The model under review builds one solid part; all positions refer to its coordinate system, in mm. Face numbers are marked on the shaded views. Round coordinates to 2 decimals unless told otherwise and drop trailing zeros. Order: outer loops, then holes, each group sorted by start corner. A loop starts at its lowest first (then second) coordinate and runs counter-clockwise, first axis right, second up. Notation, with made-up numbers: M 45,13.5 L 71,13.5 A16 cw 71,29.5 Z; hole C -6,48.5 d8. An arc over 180 degrees is marked long. Use a Markdown table: item, result. Add a question column.
1. Insertion check: P1, Ø1.5, axis at x = 83, y = 10, coming from the +Z side; P2, Ø3, axis at x = 2, z = 5, coming from the +Y side; P3, Ø3, axis at y = 27.5, z = 6, coming from the -X side; P4, Ø1, axis at x = 97.5, y = 11.5, coming from the -Z side. Each pin has a flat end and moves straight along its axis. Give the tip position at first contact, or say it passes through.
2. Consider section A-A on z = 2.75. State the section outline as (x, y) points, then the cut area to 3 significant figures.
3. To check wall thickness, follow probe 1 along Y at (x, z) = (-2.9, 0.55) (3 decimals); probe 2 along Y at (x, z) = (137.1, 0.75); probe 3 along Y at (x, z) = (67, 3.5). State the ranges of each line that lie inside material, in increasing order.
4. The part is to be moulded in two halves that separate along X. For the marked faces 1 and 2, say which applies: +X half, -X half, draft (parallel to the pull), parting line (faces both ways), or undercut.
5. Consider section C-C on x = 104.5. State the section outline as (y, z) points.
6. Consider section D-D on y = 20. State the section outline as (x, z) points, then the cut area to 3 significant figures.
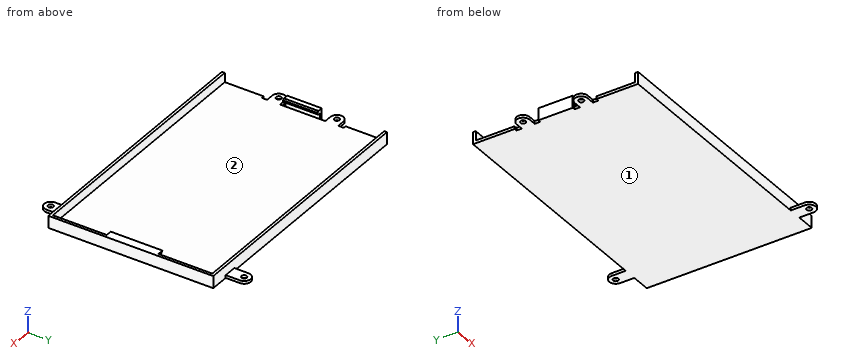
Autodesk Inventor part; units mm, degrees
ref_plane "YZ Plane" through (0, 0, 0) normal (1, 0, 0) x (0, 1, 0)
ref_plane "XZ Plane" through (0, 0, 0) normal (0, 1, 0) x (-1, 0, 0)
ref_plane "XY Plane" through (0, 0, 0) normal (0, 0, 1) x (1, 0, 0)
sketch "Sketch1" plane through (0, 0, 0) normal (0, 0, 1) x (1, 0, 0)
  line L0 (150.1, 1.6) -> (0, 1.6)
  line L1 (1.6, 24.1) -> (1.6, 71.6)
  line L2 (1.6, 24.1) -> (0, 24.1)
  line L3 (1.6, 47.85) -> (150.1, 47.85) construction
  line L4 (1.6, 71.6) -> (0, 71.6)
  line L5 (0, 71.6) -> (0, 94.1)
  line L6 (1.6, 30.975) -> (-2.9, 30.975) construction
  circle A0 centre (-2.9, 30.975) radius 1.5
  line L7 (-2.9, 27.225) -> (-2.9, 34.725) construction
  line L8 (-2.9, 27.225) -> (1.6, 27.225)
  line L9 (-2.9, 34.725) -> (1.6, 34.725)
  line L10 (1.6, 57.85) -> (0, 57.85)
  line L11 (0, 57.85) -> (0, 37.85)
  line L12 (0, 37.85) -> (1.6, 37.85)
  line L13 (0, 57.85) -> (0, 68.475) construction
  line L14 (0, 37.85) -> (0, 27.225) construction
  line L15 (0, 24.1) -> (0, 34.725) construction
  line L16 (151.7, 0) -> (0, 0)
  line L17 (151.7, 95.7) -> (0, 95.7)
  line L18 (0, 95.7) -> (0, 94.1)
  line L19 (0, 94.1) -> (150.1, 94.1)
  line L20 (137.1, 94.1) -> (137.1, 103.95) construction
  circle A1 centre (137.1, 103.95) radius 1.5
  arc A2 (140.85, 103.95) -> (133.35, 103.95) centre (137.1, 103.95) ccw
  line L21 (133.35, 103.95) -> (140.85, 103.95) construction
  line L22 (140.85, 103.95) -> (140.85, 95.7)
  line L23 (133.35, 103.95) -> (133.35, 95.7)
  line L24 (137.1, 1.6) -> (137.1, -8.25) construction
  circle A3 centre (137.1, -8.25) radius 1.5
  arc A4 (133.35, -8.25) -> (140.85, -8.25) centre (137.1, -8.25) ccw
  line L25 (133.35, -8.25) -> (140.85, -8.25) construction
  line L26 (140.85, -8.25) -> (140.85, 0)
  line L27 (133.35, -8.25) -> (133.35, 0)
  arc A5 (-2.9, 34.725) -> (-2.9, 27.225) centre (-2.9, 30.975) ccw
  line L28 (150.1, 94.1) -> (150.1, 1.6)
  line L29 (151.7, 0) -> (151.7, 95.7)
  line L30 (0, 24.1) -> (0, 0)
  line L31 (1.6, 64.725) -> (-2.9, 64.725) construction
  circle A6 centre (-2.9, 64.725) radius 1.5
  line L32 (-2.9, 68.475) -> (-2.9, 60.975) construction
  line L33 (1.6, 68.475) -> (-2.9, 68.475)
  line L34 (1.6, 60.975) -> (-2.9, 60.975)
  arc A7 (-2.9, 68.475) -> (-2.9, 60.975) centre (-2.9, 64.725) ccw
  point P0 (0, 0)
  dimension "d8" = 3
  dimension "d9" = 4.5
  dimension "d11" = 1.6
  dimension "d14" = 3
  dimension "d15" = 7.5
  dimension "d17" = 7.5
  dimension "d19" = 112.2
  dimension "d23" = 1.6
  dimension "d27" = 22.5
  dimension "d28" = 1.6
  dimension "d29" = 1.6
  dimension "d30" = 148.5
  dimension "d31" = 92.5
  dimension "d32" = 1.6
  dimension "d34" = 140
  dimension "d36" = 33.75
  dimension "d37" = 7.5
extrude "Extrusion1" add sketch "Sketch1" along normal blind 1.6
extrude "Extrusion2" add sketch "Sketch1" along normal blind 7 contours L28 L19 L18 L17 L29 L16 L30 L0 | L12 L11 L10 L1
sketch "Sketch2" plane through (150.1, 1.6, 1.6) normal (-1, 0, 0) x (0, 0, 1)
  line L0 (-1.6, -1.6) -> (-1.6, 94.1)
  line L1 (-1.6, 94.1) -> (5.4, 94.1)
  line L2 (5.4, -1.6) -> (5.4, 94.1)
  line L3 (-1.6, -1.6) -> (5.4, -1.6)
  line L4 (0, 56.25) -> (0, 36.25)
  line L5 (0, 36.25) -> (0, 33.125)
  line L6 (0, 33.125) -> (0, 25.625)
  line L7 (0, 25.625) -> (0, 22.5)
  line L8 (0, 22.5) -> (0, 0)
  line L9 (0, 0) -> (0, 92.5)
  line L10 (0, 92.5) -> (0, 70)
  line L11 (0, 70) -> (0, 66.875)
  line L12 (0, 66.875) -> (0, 59.375)
  line L13 (0, 59.375) -> (0, 56.25)
  line L14 (0, 64.625) -> (0, 61.625)
  line L15 (0, 30.875) -> (0, 27.875)
  line L16 (5.4, -1.6) -> (5.4, 94.1)
  line L17 (5.4, 61.25) -> (3.4, 61.25)
  line L18 (3.4, 61.25) -> (3.4, 31.25)
  line L19 (3.4, 31.25) -> (5.4, 31.25)
  line L20 (5.4, 31.25) -> (5.4, 61.25)
  line L21 (-1.6, -1.6) -> (-1.6, 94.1)
  line L22 (5.4, 46.25) -> (-1.6, 46.25) construction
  dimension "d42" = 2
  dimension "d43" = 30
extrude "Extrusion3" add sketch "Sketch2" along normal blind 3.5 contours L19 L18 L17 L2
chamfer "Chamfer1" distance 2 angle 45 1 edges at (146.6, 47.85, 5)
sketch "Sketch3" plane through (1.6, 37.85, 1.6) normal (1, 0, 0) x (0, 0, -1)
  line L0 (1.6, 20) -> (1.6, 0)
  line L1 (1.6, 0) -> (-5.4, 0)
  line L2 (-5.4, 20) -> (-5.4, 0)
  line L3 (1.6, 20) -> (-5.4, 20)
  line L4 (1.6, 0) -> (-5.4, 0)
  line L5 (1.6, 20) -> (-5.4, 20)
  line L6 (-5.4, 0) -> (-3.2, 0)
  line L7 (-3.2, 0) -> (-3.2, 20)
  line L8 (-3.2, 20) -> (-5.4, 20)
  line L9 (-5.4, 20) -> (-5.4, 0)
  point P0 (1.6, -37.85)
  dimension "d49" = 2.2
extrude "Extrusion4" add sketch "Sketch3" along normal blind 2 contours L7 L1 L2 L3
chamfer "Chamfer2" distance 0.75 angle 45 2 edges at (3.6, 47.85, 7) (3.6, 47.85, 4.8)
properties part number "PCB_deck"
Answer block:
| question | item | result |
|---|---|---|
| 1 | P1 | z = 1.6 |
| 1 | P2 | y = 95.7 |
| 1 | P3 | x = 150.1 |
| 1 | P4 | z = 0 |
| 2 | outline | M 0,0 L 151.7,0 L 151.7,95.7 L 0,95.7 L 0,94.1 L 150.1,94.1 L 150.1,1.6 L 0,1.6 Z; M 0,37.85 L 1.6,37.85 L 1.6,57.85 L 0,57.85 Z |
| 2 | area | 665 mm^2 |
| 3 | probe 1 | 27.225 to 29.475, 32.475 to 34.725, 60.975 to 63.225, 66.225 to 68.475 |
| 3 | probe 2 | -12 to -9.75, -6.75 to 102.45, 105.45 to 107.7 |
| 3 | probe 3 | 0 to 1.6, 94.1 to 95.7 |
| 4 | face 1 | draft |
| 4 | face 2 | undercut |
| 5 | outline | M 0,0 L 95.7,0 L 95.7,7 L 94.1,7 L 94.1,1.6 L 1.6,1.6 L 1.6,7 L 0,7 Z |
| 6 | outline | M 0,0 L 151.7,0 L 151.7,7 L 150.1,7 L 150.1,1.6 L 0,1.6 Z |
| 6 | area | 251 mm^2 |
